```python
from build123d import *

# Parameters (mm, degrees)
SKETCH1_W          = 63.5
SKETCH1_H          = 36.4998
SKETCH1_R          = 8.7503
SKETCH1_R_2        = 4.3688
EXTRUDE1_DEPTH     = 25.4
CUT_EXTRUDE1_DEPTH = 64.5
LPATTERN1_COUNT    = 2
LPATTERN1_PITCH    = 47.625


with BuildPart() as part:
    # Sketch1 → Extrude1 (new body)
    with BuildSketch(Plane.XY):
        with Locations((0, -1.1811)):
            Rectangle(SKETCH1_W, SKETCH1_H)
        Circle(SKETCH1_R, mode=Mode.SUBTRACT)
        with Locations((-23.7998, 0)):
            Circle(SKETCH1_R_2, mode=Mode.SUBTRACT)
        with Locations((23.8252, 0)):
            Circle(SKETCH1_R_2, mode=Mode.SUBTRACT)
    extrude(amount=EXTRUDE1_DEPTH)

    # Sketch2 → Cut-Extrude1 (cut, through all)
    with BuildSketch(Plane(origin=(31.75, 0, 0), x_dir=(0, 0, -1), z_dir=(1, 0, 0))):
        Polygon((0, -19.431), (-25.4, -18.099842406), (-25.4, -19.431), align=None)
    extrude(amount=-CUT_EXTRUDE1_DEPTH, mode=Mode.SUBTRACT)

    # Sketch3 → Cut-Revolve1 (revolve, cut)
    with BuildSketch(Plane(origin=(-23.7998, 0, 0), x_dir=(0, 0, -1), z_dir=(1, 0, 0)), mode=Mode.PRIVATE) as cut_revolve1_sk:
        Polygon((-10.9093, -18.859267813), (-10.9093, -8.3312), (-12.6873, -8.3312), (-12.6873, 17.0688), (-17.4498, 17.0688), (-17.4498, -18.859267813), align=None)
    cut_revolve1 = revolve(cut_revolve1_sk.sketch.rotate(Axis((-23.7998, 16.931830478, 17.4498), (0, -1, 0)), 180), axis=Axis((-23.7998, 16.931830478, 17.4498), (0, -1, 0)), mode=Mode.SUBTRACT)  # turned: the seam where the file's is

    # Sketch4 → Cut-Revolve2 (revolve, cut)
    with BuildSketch(Plane(origin=(-23.7998, 0, 0), x_dir=(0, 0, -1), z_dir=(1, 0, 0)), mode=Mode.PRIVATE) as cut_revolve2_sk:
        Polygon((-9.825313315, 17.0688), (-10.376701981, 6.547677495), (-16.908238453, 6.889980817), (-16.356849787, 17.411103322), align=None)
    cut_revolve2 = revolve(cut_revolve2_sk.sketch.rotate(Axis((-23.7998, 21.413272844, 16.14710497), (0, -0.998629535, 0.052335956)), 180), axis=Axis((-23.7998, 21.413272844, 16.14710497), (0, -0.998629535, 0.052335956)), mode=Mode.SUBTRACT)  # turned: the seam where the file's is

    # LPattern1: Cut-Revolve1, Cut-Revolve2 ×2
    with Locations(*[(i * LPATTERN1_PITCH, 0, 0) for i in range(1, LPATTERN1_COUNT)]):
        add(cut_revolve1, mode=Mode.SUBTRACT)
        add(cut_revolve2, mode=Mode.SUBTRACT)


solid = part.part
```
Input: part model. Units: mm. Frame: model coordinates. A direction names the side the tool comes from. Give positions to 0.01 mm unless a question says otherwise; leave off trailing zeros. Write each loop counter-clockwise with the first axis right and the second up, starting at its lowest first coordinate (ties: lowest second). Pieces come first, ordered by that corner, then holes. Notation, with made-up numbers: (68.25, 34.25) - (106.25, 34.25) arc R22 cw to (106.25, 42.25) - close; hole circle Ø9 at (-13.75, -35.5). An arc over 180 degrees is marked (long way). Write item = value, one per line. Start each with the question number.
1. Section query B-B, the plane y = 0. Count the separate pieces of the cut face and the enclosed holes in it, then the cut area to 4 significant figures.
2. Section query A-A, the plane x = 0. Output: boundary loops of the cut face in (y, z), then the cut area to 3 significant figures.
3. Access query for faces 1 (the flat face through (31.75, -1, 13)), 2 (the cylindrical face through (23.538, -13.522, 10.916)). Directions: +Z, -Z, +X, -X, +Y, -Y. A direction counts if a zero-diameter tool reaches every point of the face in a straight line with its end or side. Return the directions, or none.
4. First-contact query: pin 1 Ø10 at (x, z) = (-21, 14.5) entering from +Y; pin 2 Ø6.5 at (x, z) = (24.5, 19) entering from -Y; pin 3 Ø15 at (x, z) = (23.83, 17.45) entering from -Y. Flat tips, straight axial feed; report the tip coordinate or a pass-through.
5. Mould query, pull axis Z, two halves, no side actions, for faces 3 (the cylindrical face through (-24.087, -13.522, 10.916)), 4 (the cylindrical face through (27.992, 1.312, 7.668)), 5 (the flat face through (-8, -5, 0)). Classes: released by +Z, released by -Z, zero draft, split by the parting line, or undercut.
6. Ray query, L1, parallel to X at y = 4, z = 19.5; L2, parallel to X at y = 0.5, z = 10.75; L3, parallel to X at y = -10, z = 21.5. Return the intervals inside material, ascending.
7. Section query C-C, the plane x = 23. Output: boundary loops of the cut face in (y, z), then the cut area to 3 significant figures.
Check sheet entries:
q1.separate_pieces = 4
q1.enclosed_holes = 0
q1.area = 720.5 mm2
q2.outline = (-19.43, 0) - (-8.75, 0) - (-8.75, 25.4) - (-18.1, 25.4) - close; (8.75, 0) - (17.07, 0) - (17.07, 25.4) - (8.75, 25.4) - close
q2.area = 466 mm2
q3.face_1 = +Z, -Z, +X, +Y, -Y
q3.face_2 = -Y
q4.pin_1 = 17.07
q4.pin_2 = -8.33
q4.pin_3 = -18.91
q5.face_3 = undercut
q5.face_4 = zero draft
q5.face_5 = released by -Z
q6.L1 = -31.75 to -28.1, -19.5 to -7.78, 7.78 to 19.53, 28.12 to 31.75
q6.L2 = -31.75 to -28.14, -19.46 to -8.74, 8.74 to 19.49, 28.17 to 31.75
q6.L3 = -31.75 to -28.94, -18.66 to 18.69, 28.96 to 31.75
q7.outline = (-19.43, 0) - (-4.29, 0) - (-4.29, 12.76) - (-8.33, 12.76) - (-8.33, 10.96) - (-18.86, 10.96) - close; (-18.18, 23.94) - (-8.33, 23.94) - (-8.33, 22.14) - (-4.29, 22.14) - (-4.29, 25.4) - (-18.1, 25.4) - close; (4.29, 0) - (17.07, 0) - (17.07, 9.88) - (6.55, 10.43) - (6.67, 12.76) - (4.29, 12.76) - close; (4.29, 22.14) - (7.16, 22.14) - (7.23, 23.39) - (17.07, 22.87) - (17.07, 25.4) - (4.29, 25.4) - close
q7.area = 365 mm2
